CAD build for the part. Positions are in the model's coordinates, mm. Round coordinates to 2 decimals unless told otherwise and drop trailing zeros. Order: outer loops, then holes, each group sorted by start corner. A loop starts at its lowest first (then second) coordinate and runs counter-clockwise, first axis right, second up. Notation, with made-up numbers: M 28,35.5 L 55,35.5 A17 ccw 55,39.5 Z; hole C -6,66 d9. An arc over 180 degrees is marked long. Put each result on its own line as item: value.
```python
from build123d import *

# Parameters (mm, degrees)
ESQUISSE1_W                  = 76
ESQUISSE1_H                  = 100
BOSS_EXTRU_1_DEPTH           = 9
ESQUISSE2_W                  = 33.25
ESQUISSE2_H                  = 100
ESQUISSE2_W_2                = 5.5
ENL_V_MAT_EXTRU_1_DEPTH      = 7
ESQUISSE3_R                  = 1.55
ENL_V_MAT_EXTRU_2_DEPTH      = 43.75
CONG_1_R                     = 3
CONG_2_R                     = 2
ESQUISSE9_R                  = 3
BOSS_EXTRU_2_DEPTH           = 3
ESQUISSE5_R                  = 1.55
ENL_V_MAT_EXTRU_4_DEPTH      = 8
ENL_V_MAT_EXTRU_4_DEPTH_BACK = 3


with BuildPart() as part:
    # Esquisse1 → Boss.-Extru.1 (new body)
    with BuildSketch(Plane.XY):
        with Locations((38, 50)):
            Rectangle(ESQUISSE1_W, ESQUISSE1_H)
    extrude(amount=BOSS_EXTRU_1_DEPTH)

    # Esquisse2 → Enlèv. mat.-Extru.1 (cut)
    with BuildSketch(Plane(origin=(0, 0, 0), x_dir=(-1, 0, 0), z_dir=(0, 0, -1))):
        with Locations((-16.625, 50)):
            Rectangle(ESQUISSE2_W, ESQUISSE2_H)
        with Locations((-59.375, 50)):
            Rectangle(ESQUISSE2_W, ESQUISSE2_H)
        with Locations((-38, 50)):
            Rectangle(ESQUISSE2_W_2, ESQUISSE2_H)
    extrude(amount=-ENL_V_MAT_EXTRU_1_DEPTH, mode=Mode.SUBTRACT)

    # Esquisse3 → Enlèv. mat.-Extru.2 (cut, through all)
    with BuildSketch(Plane(origin=(42.75, 0, 0), x_dir=(0, 0, -1), z_dir=(1, 0, 0))):
        with Locations((-3.5, 15)):
            Circle(ESQUISSE3_R)
        with Locations((-3.5, 85)):
            Circle(ESQUISSE3_R)
    extrude(amount=-ENL_V_MAT_EXTRU_2_DEPTH, mode=Mode.SUBTRACT)

    # Congé1
    cong_1_edges = [part.edges().sort_by_distance(p)[0] for p in [
        (0, 100, 8),
        (76, 100, 8),
        (76, 0, 8),
        (0, 0, 8),
    ]]
    fillet(cong_1_edges, radius=CONG_1_R)

    # Congé2
    cong_2_edges = [part.edges().sort_by_distance(p)[0] for p in [
        (41.75, 100, 0),
        (34.25, 100, 0),
        (34.25, 0, 0),
        (41.75, 0, 0),
    ]]
    fillet(cong_2_edges, radius=CONG_2_R)

    # Esquisse9 → Boss.-Extru.2 (add)
    with BuildSketch(Plane(origin=(0, 0, 7), x_dir=(-1, 0, 0), z_dir=(0, 0, -1))):
        with Locations((-66, 92)):
            Circle(ESQUISSE9_R)
        with Locations((-10, 92)):
            Circle(ESQUISSE9_R)
        with Locations((-18, 22)):
            Circle(ESQUISSE9_R)
        with Locations((-58, 22)):
            Circle(ESQUISSE9_R)
    extrude(amount=BOSS_EXTRU_2_DEPTH)

    # Esquisse5 → Enlèv. mat.-Extru.4 (cut, two sides)
    with BuildSketch(Plane(origin=(0, 0, 7), x_dir=(-1, 0, 0), z_dir=(0, 0, -1))) as enl_v_mat_extru_4_sk:
        with Locations((-66, 92)):
            Circle(ESQUISSE5_R)
        with Locations((-58, 22)):
            Circle(ESQUISSE5_R)
        with Locations((-18, 22)):
            Circle(ESQUISSE5_R)
        with Locations((-10, 92)):
            Circle(ESQUISSE5_R)
    extrude(amount=ENL_V_MAT_EXTRU_4_DEPTH, mode=Mode.SUBTRACT)
    extrude(enl_v_mat_extru_4_sk.sketch, amount=-ENL_V_MAT_EXTRU_4_DEPTH_BACK, mode=Mode.SUBTRACT)


solid = part.part
```
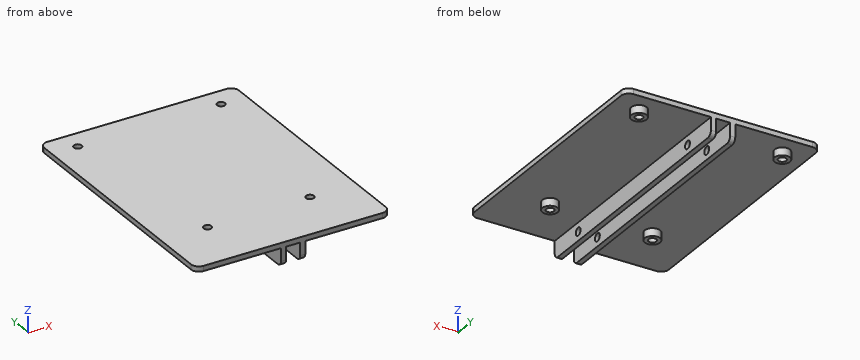
Item 1: Band-saw the part on A-A on y = 92. Give the cut face in (x, z), and give its area (3 significant figures).
Answers below:
outline: M 0,7 L 7,7 L 7,4 L 8.45,4 L 8.45,9 L 0,9 Z; M 11.55,4 L 13,4 L 13,7 L 33.25,7 L 33.25,0 L 35.25,0 L 35.25,7 L 40.75,7 L 40.75,0 L 42.75,0 L 42.75,7 L 63,7 L 63,4 L 64.45,4 L 64.45,9 L 11.55,9 Z; M 67.55,4 L 69,4 L 69,7 L 76,7 L 76,9 L 67.55,9 Z
area: 185 mm²
Item 2: Band-saw the part on D-D on x = 39. Give the cut face in (y, z), and give its area (3 significant figures).
Answers below:
outline: M 0,7 L 100,7 L 100,9 L 0,9 Z
area: 200 mm²
Item 3: Pin check, flat tips, straight feed: P1, Ø1, axis at x = 27, y = 50, coming from the -Z side; P2, Ø3.5, axis at y = 85, z = 3.5, coming from the +X side; P3, Ø5, axis at x = 10, y = 92, coming from the +Z side; P4, Ø1.5, axis at x = 60.5, z = 5.5, coming from the -Y side. Stop position of each tip, or through.
Answers below:
P1: z = 7
P2: x = 42.75
P3: z = 9
P4: y = 19.56
Item 4: Band-saw the part on C-C on y = 70.5. Give the cut face in (x, z).
Answers below:
outline: M 0,7 L 33.25,7 L 33.25,0 L 35.25,0 L 35.25,7 L 40.75,7 L 40.75,0 L 42.75,0 L 42.75,7 L 76,7 L 76,9 L 0,9 Z
Item 5: Probe line 1 along Y through (x, z) = (41.2, 3.5); line 2 along X through (y, z) = (56.5, 4.5); line 3 along Y through (x, z) = (58, 7.4). List the from-to ranges inside material, lowest first. Write a range as [from, to].
Answers below:
line 1: [0, 13.45], [16.55, 83.45], [86.55, 100]
line 2: [33.25, 35.25], [40.75, 42.75]
line 3: [0, 20.45], [23.55, 100]
Item 6: Band-saw the part on B-B on x = 18. Give the cut face in (y, z).
Answers below:
outline: M 0,7 L 19,7 L 19,4 L 20.45,4 L 20.45,9 L 0,9 Z; M 23.55,4 L 25,4 L 25,7 L 100,7 L 100,9 L 23.55,9 Z
